Work out the finished part from the listing and answer in its coordinate system (mm). Face numbers are marked on the shaded views. A direction names the side the tool comes from. Round coordinates to 2 decimals unless told otherwise and drop trailing zeros. Loops run counter-clockwise (first coordinate to the right, second up) from the corner with the lowest first, then second, coordinate; pieces in that order, holes last.
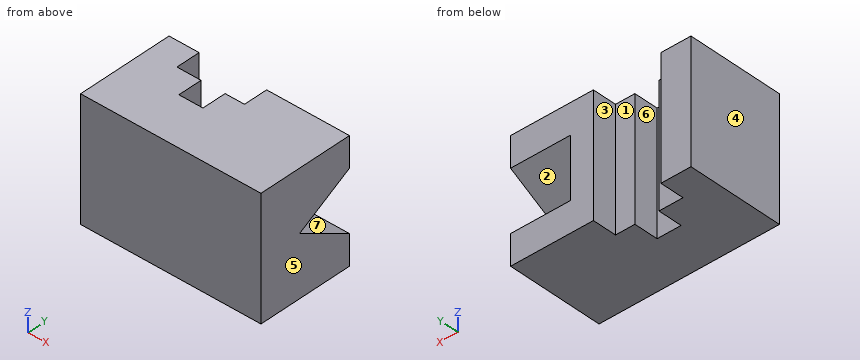
from build123d import *

# Parameters (mm, degrees)
SKETCH2_W               = 150
SKETCH2_H               = 80
BOSS_EXTRUDE1_DEPTH     = 100
CUT_EXTRUDE1_DEPTH      = 142.794426811
CUT_EXTRUDE1_DEPTH_BACK = 100
CUT_EXTRUDE2_DEPTH      = 186.671040169
CUT_EXTRUDE2_DEPTH_BACK = 50


with BuildPart() as part:
    # Sketch2 → Boss-Extrude1 (new body)
    with BuildSketch(Plane.XY):
        with Locations((15.177182909, 4.426739215)):
            Rectangle(SKETCH2_W, SKETCH2_H)
    extrude(amount=-BOSS_EXTRUDE1_DEPTH)

    # Sketch3 → Cut-Extrude1 (cut, two sides: drawn at the far end of the back side and taken through both)
    with BuildSketch(Plane.XY.offset(-CUT_EXTRUDE1_DEPTH_BACK)):
        Polygon((-409.822817091, 44.426739215), (-59.822817091, 44.426739215), (-34.822817091, 44.426739215), (-34.822817091, 24.426739215), (-14.822817091, 24.426739215), (-14.822817091, 4.426739215), (5.177182909, 4.426739215), (5.177182909, 24.426739215), (21.319701193, 24.426739215), (21.319701193, 44.426739215), (21.319701193, 394.426739215), (-419.864809368, 937.89359896), (-851.007327651, 587.89359896), align=None)
    extrude(amount=CUT_EXTRUDE1_DEPTH + CUT_EXTRUDE1_DEPTH_BACK, mode=Mode.SUBTRACT)

    # Sketch5 → Cut-Extrude2 (cut, two sides: drawn at the far end of the back side and taken through both)
    with BuildSketch(Plane(origin=(90.177182909, 0, 0), x_dir=(0, 0, -1), z_dir=(1, 0, 0)).offset(-CUT_EXTRUDE2_DEPTH_BACK)):
        Polygon((-86.366239295, 244.885969946), (25, 44.426739215), (50, -0.573260785), (75, 44.426739215), (186.366239295, 244.885969946), (186.366239295, 703.520213935), (-86.366239295, 703.520213935), align=None)
    extrude(amount=CUT_EXTRUDE2_DEPTH + CUT_EXTRUDE2_DEPTH_BACK, mode=Mode.SUBTRACT)


solid = part.part
Item 1: Section D-D, the plane y = 18 is taken. Give the vertices of the cut face in (x, z).
Item 2: Determine the mould class of the marked faces 1, 2, 3 and 4 for opening direction X: pulls with the +X half, pulls with the -X half, needs draft (parallel to the pull), parting line crosses it, or undercut.
Item 3: Section A-A, the plane z = -85.5 is taken. Give the vertices of the cut face in (x, y).
Item 4: Straight lines are drawn through the part: line 1 (X direction, y = 41.5, z = -4); line 2 (X direction, y = 12.5, z = -46.5); line 3 (Y direction, x = 4, z = -47). For each, find the intervals that lie inside material, in ascending order.
Item 5: Section B-B, the plane y = 28.5 is taken. Give the vertices of the cut face in (x, z), plus the area to 3 significant figures.
Item 6: Each of these flat-tipped pins is pushed along its axis until it touches: P1, Ø2, axis at x = 44, y = 33, coming from the +Z side; P2, Ø16, axis at x = -9, z = -62.5, coming from the +Y side. Where does it stop, or does it pass through?
Item 7: Section C-C, the plane x = 43 is taken. Give the vertices of the cut face in (y, z), plus the area to 4 significant figures.
Item 8: For the marked faces 5, 6 and 7, determine the directions among +Z, -Z, +X, -X, +Y, -Y from which every point of the face is accessible in a straight line to the end or side of a thin tool.
Answer below:
1. outline: (-59.82, -100) - (-14.82, -100) - (-14.82, 0) - (-59.82, 0) - close; (5.18, -100) - (90.18, -100) - (90.18, -60.32) - (40.18, -60.32) - (40.18, -39.68) - (90.18, -39.68) - (90.18, 0) - (5.18, 0) - close
2. face 1: undercut
2. face 2: needs draft
2. face 3: undercut
2. face 4: pulls with the -X half
3. outline: (-59.82, -35.57) - (90.18, -35.57) - (90.18, 44.43) - (21.32, 44.43) - (21.32, 24.43) - (5.18, 24.43) - (5.18, 4.43) - (-14.82, 4.43) - (-14.82, 24.43) - (-34.82, 24.43) - (-34.82, 44.43) - (-59.82, 44.43) - close
4. line 1: x = -59.82 to -34.82, 21.32 to 90.18
4. line 2: x = -59.82 to -14.82, 5.18 to 40.18
4. line 3: y = -35.57 to 4.43
5. outline: (-59.82, -100) - (-34.82, -100) - (-34.82, 0) - (-59.82, 0) - close; (21.32, -100) - (90.18, -100) - (90.18, -66.15) - (40.18, -66.15) - (40.18, -33.85) - (90.18, -33.85) - (90.18, 0) - (21.32, 0) - close
5. area: 7,770 mm2
6. P1: stops at z = 0
6. P2: stops at y = 24.43
7. outline: (-35.57, -100) - (44.43, -100) - (44.43, -75) - (-0.57, -50) - (44.43, -25) - (44.43, 0) - (-35.57, 0) - close
7. area: 6,875 mm2
8. face 5: +Z, -Z, +X, +Y, -Y
8. face 6: +Z, -Z, +Y
8. face 7: +X, +Y
